Verification items for the finished model (mm, model axes). Face numbers are marked on the shaded views. A direction names the side the tool comes from. Coordinates: 2 decimals unless noted, no trailing zeros. Write each loop counter-clockwise with the first axis right and the second up, starting at its lowest first coordinate (ties: lowest second). Pieces come first, ordered by that corner, then holes. Notation, with made-up numbers: (-10, 81) -> (41, 81) arc R18 ccw to (41, 109) -> close; hole circle Ø11 at (62.5, -28.5). An arc over 180 degrees is marked (long way). Answer in a Markdown table with one row per item.
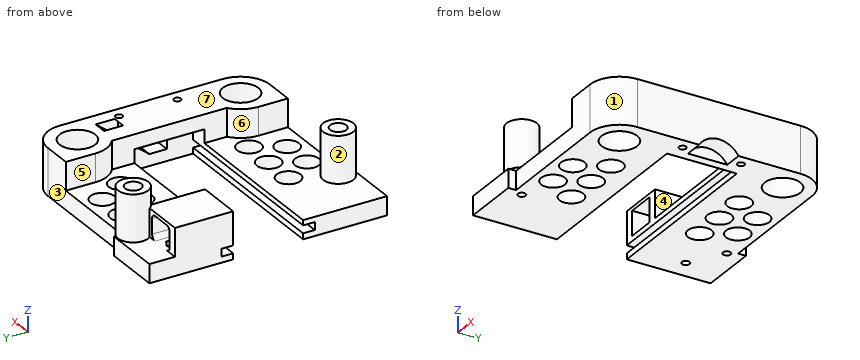
```python
from build123d import *

# Parameters (mm, degrees)
ESBO_O1_R                  = 7.65
RESSALTO_EXTRUS_O1_DEPTH   = 20
ESBO_O2_W                  = 25
ESBO_O2_H                  = 20
RESSALTO_EXTRUS_O2_DEPTH   = 51
CORTE_EXTRUS_O1_DEPTH      = 78
CORTE_EXTRUS_O4_DEPTH      = 12
ESBO_O6_R                  = 1.5
CORTE_EXTRUS_O6_DEPTH      = 13
CORTE_EXTRUS_O6_DEPTH_BACK = 9
ESBO_O7_R                  = 10
CORTE_EXTRUS_O7_DEPTH      = 8
ESBO_O9_W                  = 12.4
ESBO_O9_H                  = 10.5
CORTE_EXTRUS_O8_DEPTH      = 25
RESSALTO_EXTRUS_O3_DEPTH   = 15.5
ESBO_O12_R                 = 1.65
CORTE_EXTRUS_O9_DEPTH      = 10
CORTE_EXTRUS_O11_DEPTH     = 2
ESBO_O16_R                 = 6.5
ESBO_O16_R_2               = 3.5
RESSALTO_EXTRUS_O4_DEPTH   = 20
CORTE_EXTRUS_O13_DEPTH     = 6
ESBO_O18_R                 = 5.1
CORTE_EXTRUS_O14_DEPTH     = 10


with BuildPart() as part:
    # Esboço1 → Ressalto-extrusão1 (new body)
    with BuildSketch(Plane.XY):
        with BuildLine():
            Line((12.65, 35), (12.65, -35))
            ThreePointArc((12.65, -35), (8.944900782, -43.944900782), (0, -47.65))
            Line((0, -47.65), (-72.35, -47.65))
            Line((-72.35, -47.65), (-72.35, 47.65))
            Line((-72.35, 47.65), (0, 47.65))
            ThreePointArc((0, 47.65), (8.944900782, 43.944900782), (12.65, 35))
        make_face()
        with Locations((0, 35)):
            Circle(ESBO_O1_R, mode=Mode.SUBTRACT)
        with Locations((0, -35)):
            Circle(ESBO_O1_R, mode=Mode.SUBTRACT)
    extrude(amount=RESSALTO_EXTRUS_O1_DEPTH)

    # Esboço2 → Ressalto-extrusão2 (add, symmetric)
    with BuildSketch(Plane(origin=(0, 0, 0), x_dir=(1, 0, 0), z_dir=(0, 1, 0))):
        with Locations((-64.85, -10)):
            Rectangle(ESBO_O2_W, ESBO_O2_H)
    extrude(amount=RESSALTO_EXTRUS_O2_DEPTH, both=True)

    # Esboço3 → Corte-extrusão1 (cut)
    with BuildSketch(Plane.ZY.offset(77.35)):
        Polygon((13.8, 15), (5.8, 15), (5.8, 20), (2.5, 20), (2.5, 15), (-3, 15), (-3, -15), (2.5, -15), (2.5, -20), (5.8, -20), (5.8, -15), (13.8, -15), align=None)
    extrude(amount=-CORTE_EXTRUS_O1_DEPTH, mode=Mode.SUBTRACT)

    # Esboço4 → Corte-extrusão4 (cut)
    with BuildSketch(Plane.XY.offset(20)):
        with BuildLine():
            Line((-77.35, 40), (-57.35, 40))
            Line((-57.35, 40), (-57.35, 15))
            Line((-57.35, 15), (-77.35, 15))
            Line((-77.35, 15), (-77.35, -51))
            Line((-77.35, -51), (-52.35, -51))
            Line((-52.35, -51), (-52.35, -47.65))
            Line((-52.35, -47.65), (-12.65, -47.65))
            Line((-12.65, -47.65), (-12.65, -35))
            ThreePointArc((-12.65, -35), (-11.247221879, -29.210138171), (-7.35, -24.704369859))
            Line((-7.35, -24.704369859), (-7.35, -0.323389166))
            Line((-7.35, -0.323389166), (-7.35, 24.704369859))
            ThreePointArc((-7.35, 24.704369859), (-11.247221879, 29.210138171), (-12.65, 35))
            Line((-12.65, 35), (-12.65, 47.65))
            Line((-12.65, 47.65), (-52.35, 47.65))
            Line((-52.35, 47.65), (-52.35, 51))
            Line((-52.35, 51), (-77.35, 51))
            Line((-77.35, 51), (-77.35, 40))
        make_face()
    extrude(amount=-CORTE_EXTRUS_O4_DEPTH, mode=Mode.SUBTRACT)

    # Esboço6 → Corte-extrusão6 (cut, two sides)
    with BuildSketch(Plane.XY.offset(8)) as corte_extrus_o6_sk:
        with Locations((7.65, 12.5)):
            Circle(ESBO_O6_R)
        with Locations((7.65, -12.5)):
            Circle(ESBO_O6_R)
    extrude(amount=CORTE_EXTRUS_O6_DEPTH, mode=Mode.SUBTRACT)
    extrude(corte_extrus_o6_sk.sketch, amount=-CORTE_EXTRUS_O6_DEPTH_BACK, mode=Mode.SUBTRACT)

    # Esboço7 → Corte-extrusão7 (cut)
    with BuildSketch(Plane(origin=(12.65, 0, 0), x_dir=(0, 0, -1), z_dir=(1, 0, 0))):
        with Locations((5.349094788, 0)):
            Circle(ESBO_O7_R)
    extrude(amount=-CORTE_EXTRUS_O7_DEPTH, mode=Mode.SUBTRACT)

    # Esboço9 → Corte-extrusão8 (cut)
    with BuildSketch(Plane(origin=(0, 40, 0), x_dir=(1, 0, 0), z_dir=(0, 1, 0))):
        with Locations((-67.35, -13.25)):
            Rectangle(ESBO_O9_W, ESBO_O9_H)
    extrude(amount=-CORTE_EXTRUS_O8_DEPTH, mode=Mode.SUBTRACT)

    # Esboço10 → Ressalto-extrusão3 (add)
    with BuildSketch(Plane(origin=(0, 40, 0), x_dir=(1, 0, 0), z_dir=(0, 1, 0))):
        with BuildLine():
            Line((-71.55, -8), (-73.55, -8))
            Line((-73.55, -8), (-73.55, -10))
            ThreePointArc((-73.55, -10), (-72.964213562, -8.585786438), (-71.55, -8))
        make_face()
        with BuildLine():
            Line((-61.15, -8), (-63.15, -8))
            ThreePointArc((-63.15, -8), (-61.735786438, -8.585786438), (-61.15, -10))
            Line((-61.15, -10), (-61.15, -8))
        make_face()
        with BuildLine():
            ThreePointArc((-71.55, -18.5), (-72.964213562, -17.914213562), (-73.55, -16.5))
            Line((-73.55, -16.5), (-73.55, -18.5))
            Line((-73.55, -18.5), (-71.55, -18.5))
        make_face()
        with BuildLine():
            Line((-61.15, -18.5), (-61.15, -16.5))
            ThreePointArc((-61.15, -16.5), (-61.735786438, -17.914213562), (-63.15, -18.5))
            Line((-63.15, -18.5), (-61.15, -18.5))
        make_face()
    extrude(amount=-RESSALTO_EXTRUS_O3_DEPTH)

    # Esboço12 → Corte-extrusão9 (cut)
    with BuildSketch(Plane.XY.offset(8)):
        with Locations((-54.35, -44)):
            Circle(ESBO_O12_R)
        with Locations((-54.35, 44)):
            Circle(ESBO_O12_R)
        with Locations((-68.55, 35)):
            Circle(ESBO_O12_R)
    extrude(amount=-CORTE_EXTRUS_O9_DEPTH, mode=Mode.SUBTRACT)

    # Esboço14 → Corte-extrusão11 (cut)
    with BuildSketch(Plane.XY.offset(8)):
        Polygon((-71.45, 36.674315781), (-71.45, 33.325684219), (-68.55, 31.651368439), (-65.65, 33.325684219), (-65.65, 36.674315781), (-68.55, 38.348631561), align=None)
    extrude(amount=-CORTE_EXTRUS_O11_DEPTH, mode=Mode.SUBTRACT)

    # Esboço16 → Ressalto-extrusão4 (add)
    with BuildSketch(Plane.XY.offset(8)):
        with Locations((-54.35, 44)):
            Circle(ESBO_O16_R)
        with Locations((-54.35, 44)):
            Circle(ESBO_O16_R_2, mode=Mode.SUBTRACT)
        with Locations((-54.35, -44)):
            Circle(ESBO_O16_R)
        with Locations((-54.35, -44)):
            Circle(ESBO_O16_R_2, mode=Mode.SUBTRACT)
    extrude(amount=RESSALTO_EXTRUS_O4_DEPTH)

    # Esboço17 → Corte-extrusão13 (cut)
    with BuildSketch(Plane.ZY.offset(-0.65)):
        Polygon((11.8, 4.376686724), (11.8, -3.75), (5, -3.75), (5, 3.75), (20, 23.182890138), (20, 15), align=None)
    extrude(amount=-CORTE_EXTRUS_O13_DEPTH, mode=Mode.SUBTRACT)

    # Esboço18 → Corte-extrusão14 (cut)
    with BuildSketch(Plane.XY.offset(8)):
        with Locations((-39.35, -39.65)):
            Circle(ESBO_O18_R)
        with Locations((-32.35, -27.525644347)):
            Circle(ESBO_O18_R)
        with Locations((-46.35, -27.525644347)):
            Circle(ESBO_O18_R)
        with Locations((-25.35, -39.65)):
            Circle(ESBO_O18_R)
        with Locations((-18.35, -27.525644347)):
            Circle(ESBO_O18_R)
        with Locations((-18.35, 27.525644347)):
            Circle(ESBO_O18_R)
        with Locations((-25.35, 39.65)):
            Circle(ESBO_O18_R)
        with Locations((-46.35, 27.525644347)):
            Circle(ESBO_O18_R)
        with Locations((-32.35, 27.525644347)):
            Circle(ESBO_O18_R)
        with Locations((-39.35, 39.65)):
            Circle(ESBO_O18_R)
    extrude(amount=-CORTE_EXTRUS_O14_DEPTH, mode=Mode.SUBTRACT)


solid = part.part
```
1. Section check D-D, the plane y = 12.5. Record the boundary of the cut face in (x, z), plus the area to 3 significant figures.
Geometry says:
| item | result |
|---|---|
| outline | (-7.35, 13.8) -> (0.65, 13.8) -> (0.65, 18.07) -> (6.15, 18.07) -> (6.15, 20) -> (-7.35, 20) -> close; (0.65, 0) -> (6.15, 0) -> (6.15, 11.75) -> (0.65, 11.75) -> close; (9.15, 0) -> (12.65, 0) -> (12.65, 20) -> (9.15, 20) -> close |
| area | 195 mm^2 |
2. Section check C-C, the plane z = 22.5. Record the boundary of the cut face in (x, y), plus the area to 3 significant figures.
Geometry says:
| item | result |
|---|---|
| outline | circle Ø13 at (-54.35, -44); circle Ø13 at (-54.35, 44); hole circle Ø7 at (-54.35, -44); hole circle Ø7 at (-54.35, 44) |
| area | 188 mm^2 |
3. Section check B-B, the plane x = -2.5. Record the boundary of the cut face in (y, z), plus the area to 3 significant figures.
Geometry says:
| item | result |
|---|---|
| outline | (-47.65, 0) -> (-42.23, 0) -> (-42.23, 20) -> (-47.65, 20) -> close; (-27.77, 0) -> (-15, 0) -> (-15, 2.5) -> (-20, 2.5) -> (-20, 5.8) -> (-15, 5.8) -> (-15, 13.8) -> (15, 13.8) -> (15, 5.8) -> (20, 5.8) -> (20, 2.5) -> (15, 2.5) -> (15, 0) -> (27.77, 0) -> (27.77, 20) -> (-27.77, 20) -> close; (42.23, 0) -> (47.65, 0) -> (47.65, 20) -> (42.23, 20) -> close |
| area | 881 mm^2 |
4. Thickness scan on line 1 (Y direction, x = -39.35, z = 3.5); line 2 (X direction, y = 19, z = 15); line 3 (Y direction, x = 1, z = 19.5). Record the ranges inside material, lowest first. Write a range as from..to.
Geometry says:
| item | result |
|---|---|
| line 1 | -47.65..-44.75, -34.55..-20, 20..34.55, 44.75..47.65 |
| line 2 | -77.35..-73.55, -61.15..-57.35, -7.35..12.65 |
| line 3 | -47.61..-42.58, -27.42..14.35, 22.54..27.42, 42.58..47.61 |
5. Mould release check, pull along Y, two halves, no side actions. Record for the marked faces 1, 2 and 3: released by +Y, released by -Y, zero draft, split by the parting line, or undercut.
Geometry says:
| item | result |
|---|---|
| face 1 | released by -Y |
| face 2 | undercut |
| face 3 | released by +Y |
6. Tool access check on the marked faces 4, 5, 6 and 7. Record the directions out of +Z, -Z, +X, -X, +Y, -Y that give a thin tool (end or side, any length) a straight path to the whole face; none if there is none.
Geometry says:
| item | result |
|---|---|
| face 4 | +Z |
| face 5 | +Z, +Y, -Y |
| face 6 | +Z, -X |
| face 7 | +Z, +X, +Y, -Y |
7. Depth check by flat-ended pin: P1, Ø1, axis at x = -63, y = -26, coming from the -Z side; P2, Ø4, axis at x = 7.65, y = 12.5, coming from the +Z side; P3, Ø0.6, axis at x = -62, z = 8.5, coming from the -Y side; P4, Ø11, axis at y = 5, z = 6, coming from the -X side. Enter the tip coordinate at first touch or a pass-through.
Geometry says:
| item | result |
|---|---|
| P1 | z = 0 |
| P2 | z = 20 |
| P3 | y = 24.5 |
| P4 | x = 0.65 |
8. Section check A-A, the plane x = -32.35. Record the boundary of the cut face in (y, z).
Geometry says:
| item | result |
|---|---|
| outline | (-47.65, 0) -> (-32.63, 0) -> (-32.63, 8) -> (-47.65, 8) -> close; (-22.43, 0) -> (-15, 0) -> (-15, 2.5) -> (-20, 2.5) -> (-20, 5.8) -> (-15, 5.8) -> (-15, 8) -> (-22.43, 8) -> close; (15, 0) -> (22.43, 0) -> (22.43, 8) -> (15, 8) -> (15, 5.8) -> (20, 5.8) -> (20, 2.5) -> (15, 2.5) -> close; (32.63, 0) -> (47.65, 0) -> (47.65, 8) -> (32.63, 8) -> close |
